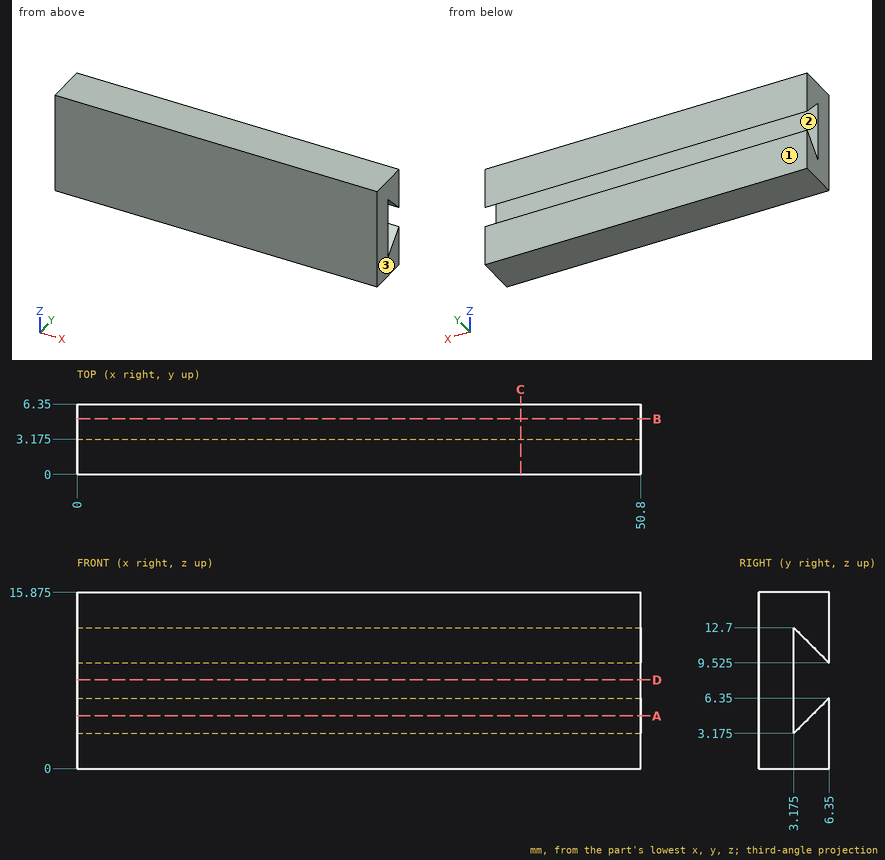
For this review, use the dimensioned drawing (mm, ordinates from the lowest corner) and the shaded views. Give positions to 0.01 mm unless a question says otherwise; leave off trailing zeros. Write each loop counter-clockwise with the first axis right and the second up, starting at its lowest first coordinate (ties: lowest second). Pieces come first, ordered by that corner, then holes.
(1) For P1, Ø1, axis at y = 5, z = 10, coming from the -X side, flat-tipped, find the tip position at first contact; note if it passes through.
(2) Consider section D-D, the plane z = 8. Give the boundary of the cut face in (x, y) (3 decimals).
(3) To check wall thickness, follow L1, parallel to Y at x = 13.5, z = 8 (3 decimals); L2, parallel to Z at x = 41, y = 4 (3 decimals); L3, parallel to Y at x = 37, z = 11.75 (3 decimals). State the ranges of each line that lie inside material, in increasing order.
(4) Consider section C-C, the plane x = 40. Give the boundary of the cut face in (y, z) (3 decimals), and give its area (3 significant figures).
(5) Consider section A-A, the plane z = 4.75. Give the boundary of the cut face in (x, y) (3 decimals).
(6) Consider section B-B, the plane y = 5. Give the boundary of the cut face in (x, z) (3 decimals), and give its area (3 significant figures).
(7) The part is to be moulded in two halves that separate along Y. For the marked faces 1, 2 and 3, say which applies: released by +Y, released by -Y, zero draft, split by the parting line, or undercut.
Returned:
1. P1: passes through
2. outline: (0, 0) - (50.8, 0) - (50.8, 3.175) - (0, 3.175) - close
3. L1: y = 0 to 3.175
3. L2: z = 0 to 4, 11.875 to 15.875
3. L3: y = 0 to 3.175, 4.125 to 6.35
4. outline: (0, 0) - (6.35, 0) - (6.35, 6.35) - (3.175, 3.175) - (3.175, 12.7) - (6.35, 9.525) - (6.35, 15.875) - (0, 15.875) - close
4. area: 80.6 mm2
5. outline: (0, 0) - (50.8, 0) - (50.8, 3.175) - (0, 3.175) - close; (0, 4.75) - (50.8, 4.75) - (50.8, 6.35) - (0, 6.35) - close
6. outline: (0, 0) - (50.8, 0) - (50.8, 5) - (0, 5) - close; (0, 10.875) - (50.8, 10.875) - (50.8, 15.875) - (0, 15.875) - close
6. area: 508 mm2
7. face 1: released by +Y
7. face 2: undercut
7. face 3: zero draft
